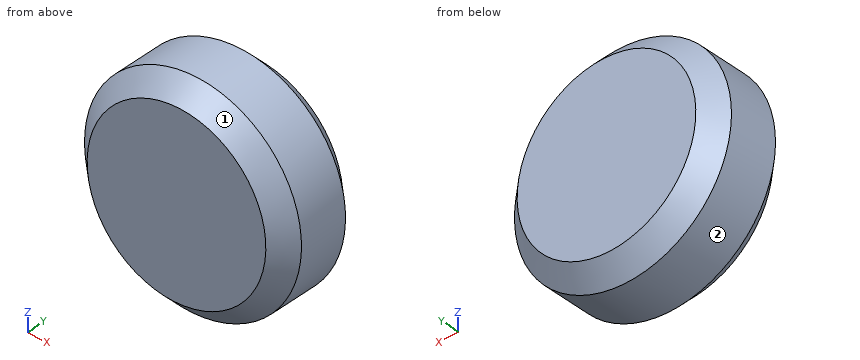
from build123d import *

# Parameters (mm, degrees)
CYLINDER012_R                = 8.5
CYLINDER012_DEPTH            = 4
FUSION006005_PLACEMENT_ANGLE = 92


with BuildPart() as cone001:
    # Cone001 → Cone001 (revolve)
    with BuildSketch(Plane(origin=(0, 0, 5.5), x_dir=(1, 0, 0), z_dir=(0, -1, 0))):
        Polygon((0, 0), (8.5, 0), (7, 1.5), (0, 1.5), align=None)
    revolve(axis=Axis((0, 0, 5.5), (0, 0, 1)))


with BuildPart() as cylinder009:
    # Cylinder012 → Cylinder012 (new body)
    with BuildSketch(Plane.XY.offset(1.5)):
        Circle(CYLINDER012_R)
    extrude(amount=CYLINDER012_DEPTH)


with BuildPart() as fusion006005:
    # Cone → Cone (revolve)
    with BuildSketch(Plane.XZ):
        Polygon((0, 0), (7, 0), (8.5, 1.5), (0, 1.5), align=None)
    revolve(axis=Axis((0, 0, 0), (0, 0, 1)))

    # Fusion006005: union Cone001, Cylinder009
    add(cone001.part)
    add(cylinder009.part)


with BuildPart() as fusion006005_1:
    # Fusion006005 placement: moved
    add(fusion006005.part.moved(Location((0, 4, 14))).rotate(Axis((0, 4, 14), (-1, 0, 0)), FUSION006005_PLACEMENT_ANGLE))


solid = fusion006005_1.part
Geometry: final body of the model. Coordinates: model frame, mm. Face numbers are marked on the shaded views. A direction names the side the tool comes from. Coordinates: 2 decimals unless noted, no trailing zeros. Use one line per item in the form item = value.
1) Pin query (flat end, axial travel): pin 1 (1 mm diameter, centred on y = 5.5, z = 20.5, fed in from -X); pin 2 (2 mm diameter, centred on x = 6, z = 13.5, fed in from -Y); pin 3 (2 mm diameter, centred on y = 8, z = 18, fed in from +X); pin 4 (8 mm diameter, centred on x = -3.5, z = 9.5, fed in from -Y). Return the tip coordinate at first contact, or that it passes through.
Solutions:
pin_1 = -5.92
pin_2 = 3.95
pin_3 = 7.9
pin_4 = 3.76
2) Ray query, L1, parallel to X at y = 6.75, z = 8.25; L2, parallel to X at y = 10, z = 12; L3, parallel to Z at x = 6.5, y = 5.5. Return the intervals inside material, ascending.
Solutions:
L1 = -6.35 to 6.35
L2 = -7.73 to 7.73
L3 = 8.47 to 19.14
3) Set-up query: the marked faces 1 and 2. Return all of +Z, -Z, +X, -X, +Y, -Y with unobstructed straight access to the full face (end or side cutting, diameter ignored); none if empty.
Solutions:
face_1 = -Y
face_2 = none
